Source: CAD feature listing. Evaluate the final solid. Frame: model axes, mm. A direction names the side the tool comes from. Coordinates: 2 decimals unless noted, no trailing zeros. Write each loop counter-clockwise with the first axis right and the second up, starting at its lowest first coordinate (ties: lowest second). Pieces come first, ordered by that corner, then holes. Notation, with made-up numbers: (-4, 25.5) - (31, 25.5) arc R22 cw to (31, 51.5) - close; hole circle Ø1 at (32.25, 38). An arc over 180 degrees is marked (long way). One line per question, with ' | ' between items.
from build123d import *

# Parameters (mm, degrees)
F0_W     = 50
F0_H     = 50
F0_R     = 5
F1_DEPTH = 3
F2_DEPTH = 5


with BuildPart() as f1:
    # F0 (on Top) → F1 (new body)
    with BuildSketch(Plane.XY):
        Rectangle(F0_W, F0_H)
        with Locations((-15, -15)):
            Circle(F0_R, mode=Mode.SUBTRACT)
        with Locations((0, -15)):
            Circle(F0_R, mode=Mode.SUBTRACT)
        with Locations((15, -15)):
            Circle(F0_R, mode=Mode.SUBTRACT)
        with Locations((-15, 0)):
            Circle(F0_R, mode=Mode.SUBTRACT)
        with Locations((-15, 15)):
            Circle(F0_R, mode=Mode.SUBTRACT)
        Circle(F0_R, mode=Mode.SUBTRACT)
        with Locations((15, 0)):
            Circle(F0_R, mode=Mode.SUBTRACT)
        with Locations((0, 15)):
            Circle(F0_R, mode=Mode.SUBTRACT)
        with Locations((15, 15)):
            Circle(F0_R, mode=Mode.SUBTRACT)
        with Locations((-15, 15)):
            Circle(F0_R)
        with Locations((0, 15)):
            Circle(F0_R)
        with Locations((15, 15)):
            Circle(F0_R)
        with Locations((15, 0)):
            Circle(F0_R)
        Circle(F0_R)
        with Locations((-15, 0)):
            Circle(F0_R)
        with Locations((-15, -15)):
            Circle(F0_R)
        with Locations((0, -15)):
            Circle(F0_R)
        with Locations((15, -15)):
            Circle(F0_R)
    extrude(amount=F1_DEPTH)

    # F0 (on Top) → F2 (join)
    with BuildSketch(Plane.XY):
        Rectangle(F0_W, F0_H)
        with Locations((-15, -15)):
            Circle(F0_R, mode=Mode.SUBTRACT)
        with Locations((0, -15)):
            Circle(F0_R, mode=Mode.SUBTRACT)
        with Locations((15, -15)):
            Circle(F0_R, mode=Mode.SUBTRACT)
        with Locations((-15, 0)):
            Circle(F0_R, mode=Mode.SUBTRACT)
        with Locations((-15, 15)):
            Circle(F0_R, mode=Mode.SUBTRACT)
        Circle(F0_R, mode=Mode.SUBTRACT)
        with Locations((15, 0)):
            Circle(F0_R, mode=Mode.SUBTRACT)
        with Locations((0, 15)):
            Circle(F0_R, mode=Mode.SUBTRACT)
        with Locations((15, 15)):
            Circle(F0_R, mode=Mode.SUBTRACT)
    extrude(amount=F2_DEPTH)


solid = f1.part
Item 1: Cut plane A-A on y = -19. Return loops of the section in (x, z), and give its area (3 significant figures).
Check sheet entries:
outline: (-25, 0) - (25, 0) - (25, 5) - (18, 5) - (18, 3) - (12, 3) - (12, 5) - (3, 5) - (3, 3) - (-3, 3) - (-3, 5) - (-12, 5) - (-12, 3) - (-18, 3) - (-18, 5) - (-25, 5) - close | area: 214 mm²
Item 2: Cut plane B-B on x = 15. Return loops of the section in (y, z).
Check sheet entries:
outline: (-25, 0) - (25, 0) - (25, 5) - (20, 5) - (20, 3) - (10, 3) - (10, 5) - (5, 5) - (5, 3) - (-5, 3) - (-5, 5) - (-10, 5) - (-10, 3) - (-20, 3) - (-20, 5) - (-25, 5) - close
Item 3: Pin query (flat end, axial travel): pin 1 Ø16 at (x, y) = (-15, -15) entering from -Z; pin 2 Ø3 at (x, y) = (15, -17) entering from +Z. Return the tip coordinate at first contact, or that it passes through.
Check sheet entries:
pin 1: z = 0 | pin 2: z = 3
Item 4: Ray query, line 1 along X through (y, z) = (0, 3.7); line 2 along X through (y, z) = (-18.5, 4.65). Return the intervals inside material, ascending. Write a range as [from, to].
Check sheet entries:
line 1: [-25, -20], [-10, -5], [5, 10], [20, 25] | line 2: [-25, -18.57], [-11.43, -3.57], [3.57, 11.43], [18.57, 25]
Item 5: Access query for faces 1 (the face through (0, 6, 5)), 2 (the face through (0, -15, 3)). Directions: +Z, -Z, +X, -X, +Y, -Y. A direction counts if a zero-diameter tool reaches every point of the face in a straight line with its end or side. Return the directions, or none.
Check sheet entries:
face 1: +Z, +X, -X, +Y, -Y | face 2: +Z
Item 6: Mould query, pull axis Y, two halves, no side actions, for faces 3 (the face through (-25, 0, 2)), 4 (the face through (17.307, -19.436, 3.986)), 5 (the face through (0, -25, 2)). Classes: pulls with the +Y half, pulls with the -Y half, needs draft (parallel to the pull), parting line crosses it, or undercut.
Check sheet entries:
face 3: needs draft | face 4: undercut | face 5: pulls with the -Y half
